```python
from build123d import *

# Parameters (mm, degrees)
F0_W     = 19.304
F0_H     = 76.454
F1_DEPTH = 19.05
F2_R     = 101.6
F3_R     = 1270
F5_DEPTH = 187.96


with BuildPart() as f1:
    # F0 (on Top) → F1 (new body)
    with BuildSketch(Plane.XY):
        Polygon((-304.8, 0), (0, 0), (304.8, 0), (406.4, 1270), (373.888, 1676.4), (0, 1676.4), (-373.888, 1676.4), (-406.4, 1270), align=None)
        with Locations((-263.652, 1251.83646)):
            Rectangle(F0_W, F0_H, mode=Mode.SUBTRACT)
        with Locations((-263.652, 1492.88246)):
            Rectangle(F0_W, F0_H, mode=Mode.SUBTRACT)
        with Locations((263.652, 1251.83646)):
            Rectangle(F0_W, F0_H, mode=Mode.SUBTRACT)
        with Locations((263.652, 1492.88246)):
            Rectangle(F0_W, F0_H, mode=Mode.SUBTRACT)
    extrude(amount=F1_DEPTH)

    # F2
    f2_edges = [f1.edges().sort_by_distance(p)[0] for p in [
        (-304.8, 0, 9.525),
        (304.8, 0, 9.525),
        (-373.888, 1676.4, 9.525),
        (373.888, 1676.4, 9.525),
    ]]
    fillet(f2_edges, radius=F2_R)

    # F3
    f3_edges = [f1.edges().sort_by_distance(p)[0] for p in [
        (-406.4, 1270, 9.525),
        (406.4, 1270, 9.525),
    ]]
    fillet(f3_edges, radius=F3_R)

    # F4 (on face) → F5 (cut)
    with BuildSketch(Plane.XY.offset(19.05)):
        Polygon((-217.7893998235, 182.3674977936), (-241.0829792523, 473.537240654), (-342.0368743239, 465.4609290482), (-318.743294895, 174.2911861878), align=None)
        Polygon((217.7893998235, 182.3674977936), (318.743294895, 174.2911861878), (342.0368743239, 465.4609290482), (241.0829792523, 473.537240654), align=None)
    extrude(amount=-F5_DEPTH, mode=Mode.SUBTRACT)


solid = f1.part
```
Verification items for the finished model (mm, model axes). Give positions to 0.01 mm unless a question says otherwise; leave off trailing zeros. Order: outer loops, then holes, each group sorted by start corner. A loop starts at its lowest first (then second) coordinate and runs counter-clockwise, first axis right, second up. Notation, with made-up numbers: (-32.75, -9.75) - (-5.75, -9.75) arc R38 ccw to (-5.75, 28.25) - close; hole circle Ø4 at (76, 38.5). An arc over 180 degrees is marked (long way). Answer as CSV lines item,"result". Start each with the question number.
Item 1: Section check B-B, the plane y = 1071. Record the boundary of the cut face in (x, z).
Item 2: Section check A-A, the plane y = 1506. Record the boundary of the cut face in (x, z).
Item 3: Section check D-D, the plane y = 1259. Record the boundary of the cut face in (x, z).
Item 4: Material ranges on L1, parallel to X at y = 1214.5, z = 6.5; L2, parallel to Y at x = 266, z = 6.5; L3, parallel to X at y = 1232.5, z = 2.75, recorded low to high.
Item 5: Section check C-C, the plane z = 16. State how many separate pieces and enclosed holes the cut face has, plus the area to 3 significant figures.
Item 6: Mould release check, pull along X, two halves, no side actions. Record for faces 1 (the face through (369.774, 812.169, 9.392)), 2 (the face through (-370.56, 822.02, 9.39)), 3 (the face through (-6, 850, 19.05)): released by +X, released by -X, zero draft, split by the parting line, or undercut.
Item 7: Gauge pin test, flat ends, axial feed: pin 1 (5.5 mm diameter, centred on x = -265.5, z = 12.5, fed in from -Y); pin 2 (9.5 mm diameter, centred on x = -262.5, z = 12, fed in from -Y); pin 3 (9.5 mm diameter, centred on y = 1492, z = 6.5, fed in from -X). Record the tip position at first contact, or that the pin passes through.
Filled in:
1,outline,"(-390.48, 0) - (390.48, 0) - (390.48, 19.05) - (-390.48, 19.05) - close"
2,outline,"(-387.52, 0) - (-273.3, 0) - (-273.3, 19.05) - (-387.52, 19.05) - close; (-254, 0) - (254, 0) - (254, 19.05) - (-254, 19.05) - close; (273.3, 0) - (387.52, 0) - (387.52, 19.05) - (273.3, 19.05) - close"
3,outline,"(-402.29, 0) - (-273.3, 0) - (-273.3, 19.05) - (-402.29, 19.05) - close; (-254, 0) - (254, 0) - (254, 19.05) - (-254, 19.05) - close; (273.3, 0) - (402.29, 0) - (402.29, 19.05) - (273.3, 19.05) - close"
4,L1,"-401.13 to -273.3, -254 to 254, 273.3 to 401.13"
4,L2,"16.17 to 178.51, 471.54 to 1213.61, 1290.06 to 1454.66, 1531.11 to 1676.4"
4,L3,"-401.79 to -273.3, -254 to 254, 273.3 to 401.79"
5,separate pieces,"1"
5,enclosed holes,"4"
5,area,"1,150,000 mm^2"
6,face 1,"released by +X"
6,face 2,"released by -X"
6,face 3,"zero draft"
7,pin 1,"y = 14.17"
7,pin 2,"y = 11.39"
7,pin 3,"x = -389.02"
